```python
from build123d import *

# Parameters (mm, degrees)
F0_W     = 19.05
F0_H     = 19.05
F1_DEPTH = 19.05
F3_DEPTH = 1.27
F5_DEPTH = 1.27


with BuildPart() as f1:
    # F0 (on Front) → F1 (new body)
    with BuildSketch(Plane.XZ):
        with Locations((-42.3251483589, 44.0142245242)):
            Rectangle(F0_W, F0_H)
    extrude(amount=F1_DEPTH)

    # F2 (on face) → F3 (join)
    with BuildSketch(Plane.XY.offset(53.5392245242)):
        with BuildLine():
            Line((-45.5001483589, -19.05), (-39.1501483589, -19.05))
            ThreePointArc((-39.1501483589, -19.05), (-42.3251483589, -15.875), (-45.5001483589, -19.05))
        make_face()
    extrude(amount=F3_DEPTH)

    # F4 (on face) → F5 (join)
    with BuildSketch(Plane.XY.offset(54.8092245242)):
        with BuildLine():
            Line((-45.5001483589, -19.05), (-39.1501483589, -19.05))
            ThreePointArc((-39.1501483589, -19.05), (-42.3251483589, -15.875), (-45.5001483589, -19.05))
        make_face()
        with BuildLine():
            Line((-39.1501483589, -19.05), (-35.9751483589, -19.05))
            ThreePointArc((-35.9751483589, -19.05), (-42.3251483589, -12.7), (-48.6751483589, -19.05))
            Line((-48.6751483589, -19.05), (-45.5001483589, -19.05))
            ThreePointArc((-45.5001483589, -19.05), (-42.3251483589, -15.875), (-39.1501483589, -19.05))
        make_face()
    extrude(amount=F5_DEPTH)


solid = f1.part
```
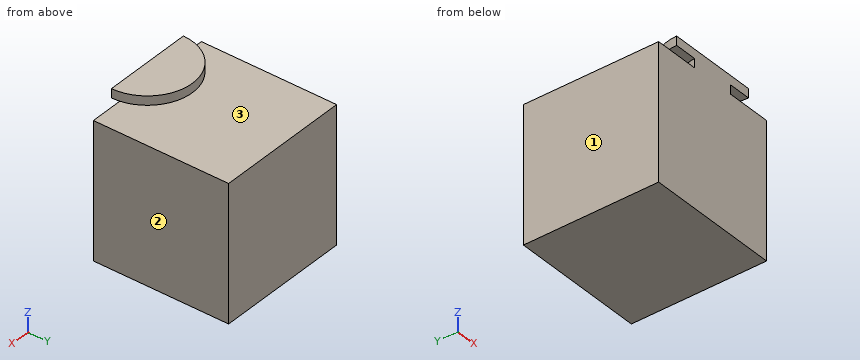
Verification items for the finished model (mm, model axes). Face numbers are marked on the shaded views. Give positions to 0.01 mm unless a question says otherwise; leave off trailing zeros. Order: outer loops, then holes, each group sorted by start corner. A loop starts at its lowest first (then second) coordinate and runs counter-clockwise, first axis right, second up. Notation, with made-up numbers: (31, -20.75) -> (58, -20.75) arc R15 cw to (58, -3.75) -> close; hole circle Ø10 at (7, 81). An arc over 180 degrees is marked (long way). One line per item, written item: value.
(1) Gauge pin test, flat end, axial feed: pin 1 (3 mm diameter, centred on x = -38.5, y = -6.5, fed in from +Z). Record the tip position at first contact, or that the pin passes through.
Final values:
pin 1: z = 53.54
(2) Scan lines: line 1 along Z through (x, y) = (-38, -16.5); line 2 along Z through (x, y) = (-46, -6.5). Record each from-to range of solid material in increasing order. Write a range as [from, to].
Final values:
line 1: [34.49, 53.54], [54.81, 56.08]
line 2: [34.49, 53.54]
(3) Sectioned sample at B-B on z = 54. Record the cut outline in (x, y) (3 decimals).
Final values:
outline: (-45.5, -19.05) -> (-39.15, -19.05) arc R3.175 ccw to start
(4) Draft check along X on the marked faces 1, 2 and 3. Enter one of: pulls with the +X half, pulls with the -X half, needs draft (parallel to the pull), parting line crosses it, or undercut.
Final values:
face 1: pulls with the -X half
face 2: pulls with the +X half
face 3: needs draft
(5) Sectioned sample at D-D on y = -10.5. Record the cut outline in (x, z).
Final values:
outline: (-51.85, 34.49) -> (-32.8, 34.49) -> (-32.8, 53.54) -> (-51.85, 53.54) -> close
(6) Sectioned sample at C-C on y = -16.25. Record the cut outline in (x, z).
Final values:
outline: (-51.85, 34.49) -> (-32.8, 34.49) -> (-32.8, 53.54) -> (-40.83, 53.54) -> (-40.83, 54.81) -> (-36.63, 54.81) -> (-36.63, 56.08) -> (-48.02, 56.08) -> (-48.02, 54.81) -> (-43.82, 54.81) -> (-43.82, 53.54) -> (-51.85, 53.54) -> close
(7) Sectioned sample at A-A on x = -39.5. Record the cut outline in (y, z).
Final values:
outline: (-19.05, 34.49) -> (0, 34.49) -> (0, 53.54) -> (-17.6, 53.54) -> (-17.6, 54.81) -> (-13.36, 54.81) -> (-13.36, 56.08) -> (-19.05, 56.08) -> close
